from build123d import *

# Parameters (mm, degrees)
BOSS_EXTRUDE1_DEPTH = 6
CUT_EXTRUDE1_DEPTH  = 270.845326067
SKETCH3_R           = 5
CUT_EXTRUDE2_DEPTH  = 1
FILLET1_R           = 5


with BuildPart() as part:
    # Sketch1 → Boss-Extrude1 (new body)
    with BuildSketch(Plane(origin=(0, 0, 0), x_dir=(1, 0, 0), z_dir=(0, 1, 0))):
        Polygon((0, -180.5), (200.5, -180.5), (200.5, -120.5), (180, -120.5), (180, 0), (180, 120.5), (200.5, 120.5), (200.5, 180.5), (0, 180.5), (-200.5, 180.5), (-200.5, 120.5), (-180, 120.5), (-180, 0), (-180, -120.5), (-200.5, -120.5), (-200.5, -180.5), align=None)
    extrude(amount=BOSS_EXTRUDE1_DEPTH)

    # Sketch2 → Cut-Extrude1 (cut, through all)
    with BuildSketch(Plane(origin=(0, 6, 0), x_dir=(1, 0, 0), z_dir=(0, 1, 0))):
        with BuildLine():
            Line((187.4, -150.5), (187.4, -144.770831301))
            ThreePointArc((187.4, -144.770831301), (190, -135.5), (192.6, -144.770831301))
            Line((192.6, -144.770831301), (192.6, -150.5))
            ThreePointArc((192.6, -150.5), (190, -153.1), (187.4, -150.5))
        make_face()
        with BuildLine():
            Line((187.4, 150.5), (187.4, 156.229168699))
            ThreePointArc((187.4, 156.229168699), (190, 165.5), (192.6, 156.229168699))
            Line((192.6, 156.229168699), (192.6, 150.5))
            ThreePointArc((192.6, 150.5), (190, 147.9), (187.4, 150.5))
        make_face()
    cut_extrude1 = extrude(amount=-CUT_EXTRUDE1_DEPTH, mode=Mode.SUBTRACT)

    # Sketch3 → Cut-Extrude2 (cut)
    with BuildSketch(Plane(origin=(0, 6, 0), x_dir=(1, 0, 0), z_dir=(0, 1, 0))):
        with Locations((190, 150.5)):
            Circle(SKETCH3_R)
        with Locations((190, -150.5)):
            Circle(SKETCH3_R)
    cut_extrude2 = extrude(amount=-CUT_EXTRUDE2_DEPTH, mode=Mode.SUBTRACT)

    # Mirror1: Cut-Extrude1, Cut-Extrude2 across plane
    add(cut_extrude1.mirror(Plane(origin=(0, 0, 0), x_dir=(0, 0, 1), z_dir=(1, 0, 0))), mode=Mode.SUBTRACT)
    add(cut_extrude2.mirror(Plane(origin=(0, 0, 0), x_dir=(0, 0, 1), z_dir=(1, 0, 0))), mode=Mode.SUBTRACT)

    # Fillet1
    fillet1_edges = [part.edges().sort_by_distance(p)[0] for p in [
        (-200.5, 3, 180.5),
        (-200.5, 3, 120.5),
        (-180, 3, 120.5),
        (-180, 3, -120.5),
        (-200.5, 3, -120.5),
        (-200.5, 3, -180.5),
        (200.5, 3, -180.5),
        (200.5, 3, -120.5),
        (180, 3, -120.5),
        (180, 3, 120.5),
        (200.5, 3, 120.5),
        (200.5, 3, 180.5),
    ]]
    fillet(fillet1_edges, radius=FILLET1_R)


solid = part.part
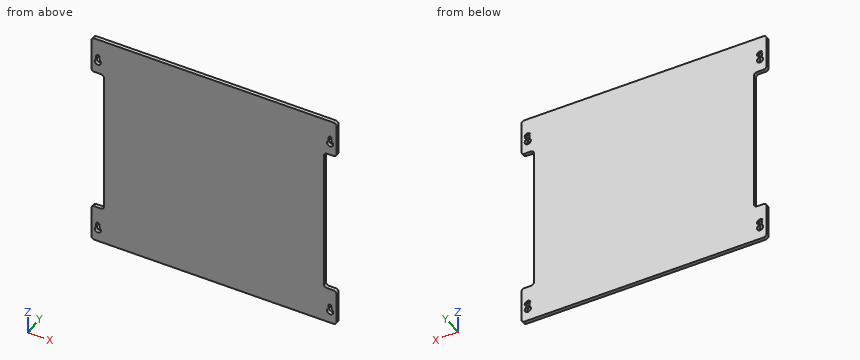
Read the model definition and answer for the solid it produces. Units are mm, in the model's axes. Coordinates: 2 decimals unless noted, no trailing zeros. Loops run counter-clockwise (first coordinate to the right, second up) from the corner with the lowest first, then second, coordinate; pieces in that order, holes last.
Q1. The part is cut by section A-A on y = 3.9. Give the number of separate pieces and of enclosed holes in the cut face, and give its area (3 significant figures).
Q2. Consider probe 1 along X at (y, z) = (5.4, 150.5); probe 2 along X at (y, z) = (2.7, -152.5); probe 3 along Z at (x, y) = (-190, 4.55). Determine where each line is inside the solid, lowest interval first.
Q3. Each of these flat-tipped pins is pushed along its axis until it touches: pin 1 Ø9 at (x, z) = (190, -150.5) entering from +Y; pin 2 Ø8 at (x, z) = (190, -160.5) entering from +Y. Where does it stop, or does it pass through?
Q4. The part is cut by section B-B on z = -86.5. Write down the section's boundary in (x, y).
Results below:
1. separate pieces: 1
1. enclosed holes: 4
1. area: 134,000 mm2
2. probe 1: x = -200.5 to -195, -185 to 185, 195 to 200.5
2. probe 2: x = -200.5 to -192.6, -187.4 to 187.4, 192.6 to 200.5
2. probe 3: z = -180.5 to -165.5, -147.9 to -120.5, 120.5 to 135.5, 153.1 to 180.5
3. pin 1: stops at y = 5
3. pin 2: passes through
4. outline: (-180, 0) - (180, 0) - (180, 6) - (-180, 6) - close
